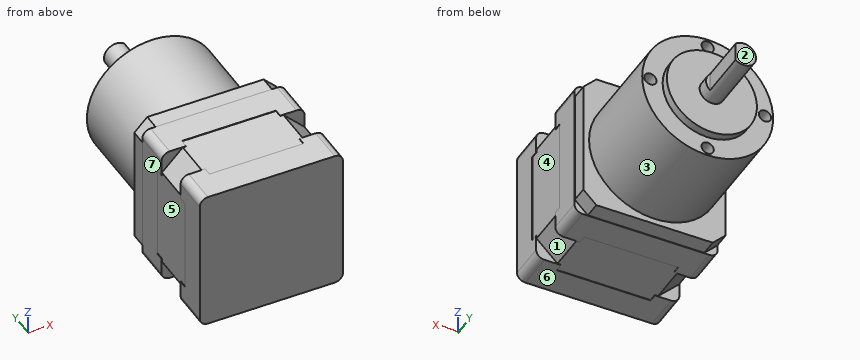
Autodesk Inventor part; units mm, degrees
ref_plane "YZ Plane" through (0, 0, 0) normal (1, 0, 0) x (0, 1, 0)
ref_plane "XZ Plane" through (0, 0, 0) normal (0, 1, 0) x (-1, 0, 0)
ref_plane "XY Plane" through (0, 0, 0) normal (0, 0, 1) x (1, 0, 0)
sketch "Sketch1" plane through (0, 0, 0) normal (0, 1, 0) x (-1, 0, 0)
  circle A0 centre (0, 0) radius 3
  dimension "d0" = 6
extrude "Extrusion1" add sketch "Sketch1" against normal blind 15
sketch "Sketch2" plane through (0, -15, 0) normal (0, -1, 0) x (1, 0, 0)
  circle A0 centre (0, 0) radius 11
  dimension "d3" = 22
extrude "Extrusion2" add sketch "Sketch2" along normal blind 2
sketch "Sketch3" plane through (0, -17, 0) normal (0, -1, 0) x (1, 0, 0)
  circle A0 centre (0, 0) radius 16
  dimension "d6" = 32
extrude "Extrusion3" add sketch "Sketch3" along normal blind 29
sketch "Sketch4" plane through (0, -46, 0) normal (0, -1, 0) x (1, 0, 0)
  line L0 (-17.4, 17.4) -> (17.4, 17.4)
  line L1 (17.4, 17.4) -> (17.4, -17.4)
  line L2 (17.4, -17.4) -> (-17.4, -17.4)
  line L3 (-17.4, -17.4) -> (-17.4, 17.4)
  line L4 (-17.4, 17.4) -> (17.4, -17.4) construction
  line L5 (17.4, 17.4) -> (-17.4, -17.4) construction
  point P0 (0, 0)
  dimension "d9" = 34.8
  dimension "d10" = 34.8
extrude "Extrusion4" add sketch "Sketch4" against normal blind 4
chamfer "Chamfer1" distance 3.175 angle 45 4 edges at (17.4, -44, 17.4) (17.4, -44, -17.4) (-17.4, -44, 17.4) (-17.4, -44, -17.4)
sketch "Sketch5" plane through (0, -46, 0) normal (0, -1, 0) x (1, 0, 0)
  line L0 (17.5, -17.5) -> (-17.5, -17.5)
  line L1 (-17.5, -17.5) -> (-17.5, 17.5)
  line L2 (-17.5, 17.5) -> (17.5, 17.5)
  line L3 (17.5, 17.5) -> (17.5, -17.5)
  line L4 (17.5, -17.5) -> (-17.5, 17.5) construction
  line L5 (-17.5, -17.5) -> (17.5, 17.5) construction
  point P0 (0, 0)
  dimension "d16" = 35
  dimension "d17" = 35
extrude "Extrusion5" add sketch "Sketch5" along normal blind 7
sketch "Sketch6" plane through (0, -53, 0) normal (0, -1, 0) x (1, 0, 0)
  line L0 (-17.5, 17.5) -> (-17.5, -17.5)
  line L1 (-17.5, -17.5) -> (17.5, -17.5)
  line L2 (17.5, -17.5) -> (17.5, 17.5)
  line L3 (17.5, 17.5) -> (-17.5, 17.5)
  line L4 (11.5, 17.5) -> (17.5, 17.5)
  line L5 (17.5, 17.5) -> (17.5, 11.5)
  line L6 (17.5, 11.5) -> (11.5, 11.5)
  line L7 (11.5, 11.5) -> (11.5, 17.5)
  circle A0 centre (0, 0) radius 16
  circle A1 centre (0, 0) radius 16
  line L8 (-17.5, 17.5) -> (-11.5, 17.5)
  line L9 (-17.5, 11.5) -> (-17.5, 17.5)
  line L10 (-11.5, 11.5) -> (-17.5, 11.5)
  line L11 (-11.5, 17.5) -> (-11.5, 11.5)
  line L12 (-17.5, -17.5) -> (-17.5, -11.5)
  line L13 (-11.5, -17.5) -> (-17.5, -17.5)
  line L14 (-11.5, -11.5) -> (-11.5, -17.5)
  line L15 (-17.5, -11.5) -> (-11.5, -11.5)
  line L16 (17.5, -17.5) -> (11.5, -17.5)
  line L17 (17.5, -11.5) -> (17.5, -17.5)
  line L18 (11.5, -11.5) -> (17.5, -11.5)
  line L19 (11.5, -17.5) -> (11.5, -11.5)
  dimension "d43" = 6
  dimension "d44" = 6
  dimension "d47" = 360
extrude "Extrusion6" add sketch "Sketch6" along normal blind 2 contours L3 L11 L10 L0 | L15 L14 L1 L0 | L3 L2 L6 L7 | L19 L18 L2 L1
fillet "Fillet2" radius 2 4 edges at (17.5, -50.5, -17.5) (-17.5, -50.5, -17.5) (-17.5, -50.5, 17.5) (17.5, -50.5, 17.5)
sketch "Sketch7" plane through (0, -53, 0) normal (0, -1, 0) x (1, 0, 0)
  line L0 (-12.2985, -17.4) -> (12.2985, -17.4)
  line L1 (17.4, -12.2985) -> (17.4, 12.2985)
  line L2 (12.2985, 17.4) -> (-12.2985, 17.4)
  line L3 (-17.4, 12.2985) -> (-17.4, -12.2985)
  line L4 (-17.4, -17.4) -> (17.4, 17.4) construction
  line L5 (17.4, -17.4) -> (-17.4, 17.4) construction
  line L6 (-17.4, -12.2985) -> (-12.2985, -17.4)
  line L7 (12.2985, -17.4) -> (17.4, -12.2985)
  line L8 (17.4, 12.2985) -> (12.2985, 17.4)
  line L9 (-12.2985, 17.4) -> (-17.4, 12.2985)
  point P0 (0, 0)
  dimension "d31" = 34.8
  dimension "d32" = 34.8
  dimension "d67" = 42
  dimension "d68" = 42
extrude "Extrusion7" add sketch "Sketch7" along normal blind 6.5
mirror "Mirror1" about plane through (0, -59.5, 0) normal (0, -1, 0) of "Extrusion6", "Extrusion5", "Fillet2", "Extrusion7"
sketch "Sketch8" plane through (0, 0, 0) normal (0, 1, 0) x (1, 0, 0)
  circle A0 centre (0, 0) radius 3
  line L0 (2, 2.2361) -> (2, -2.2361)
  dimension "d50" = 2
extrude "Extrusion8" cut sketch "Sketch8" against normal blind 12 contours A0 L0 picked at (2.1409, -0.5898)
fillet "Fillet3" radius 0.1 1 edges at (2, -12, 0)
sketch "Sketch9" plane through (0, -17, 0) normal (0, 1, 0) x (1, 0, 0)
  circle A0 centre (0, 0) radius 11
  circle A1 centre (0, 0) radius 3
  line L0 (0, 0) -> (0, -14) construction
  circle A2 centre (0, -14) radius 1.5
  dimension "d54" = 14
  dimension "d55" = 3
extrude "Extrusion9" cut sketch "Sketch9" against normal blind 5 contours A2
thread "Thread1"
pattern_circular "Circular Pattern1" count 4 over 360 about axis through (0, -17, 0) along (0, -1, 0) of "Extrusion9"
properties part number "gearedstepper"
Input: part model. Units: mm. Frame: model coordinates. Face numbers are marked on the shaded views. A direction names the side the tool comes from. Round coordinates to 2 decimals unless told otherwise and drop trailing zeros. Loops run counter-clockwise (first coordinate to the right, second up) from the corner with the lowest first, then second, coordinate; pieces in that order, holes last. Notation, with made-up numbers: (-3, 48) -> (21, 48) arc R32 ccw to (21, 76) -> close; hole circle Ø8 at (86, 41.5). An arc over 180 degrees is marked (long way). One line per item, written item: value.
(1) Section C-C (z = 7). Return the cut outline in (x, y).
Geometry check:
outline: (-17.5, -73) -> (17.5, -73) -> (17.5, -66) -> (17.4, -66) -> (17.4, -53) -> (17.5, -53) -> (17.5, -46) -> (17.4, -46) -> (17.4, -42) -> (14.39, -42) -> (14.39, -17) -> (8.49, -17) -> (8.49, -15) -> (-8.49, -15) -> (-8.49, -17) -> (-14.39, -17) -> (-14.39, -42) -> (-17.4, -42) -> (-17.4, -46) -> (-17.5, -46) -> (-17.5, -53) -> (-17.4, -53) -> (-17.4, -66) -> (-17.5, -66) -> close
(2) Pin query (flat end, axial travel): pin 1 (3 mm diameter, centred on y = -44, z = -4.5, fed in from -X); pin 2 (3.5 mm diameter, centred on y = -7, z = 0, fed in from +X); pin 3 (1 mm diameter, centred on y = -18.5, z = 1, fed in from +X). Return the tip coordinate at first contact, or that it passes through.
Geometry check:
pin 1: x = -17.4
pin 2: x = 2
pin 3: x = 15.99
(3) Mould query, pull axis Z, two halves, no side actions, for the marked faces 4, 5, 6 and 7. Classes: pulls with the +Z half, pulls with the -Z half, needs draft (parallel to the pull), parting line crosses it, or undercut.
Geometry check:
face 4: undercut
face 5: undercut
face 6: pulls with the -Z half
face 7: needs draft
(4) Section A-A (y = -62.5). Return the cut outline in (x, z), plus the area to 3 significant figures.
Geometry check:
outline: (-17.4, -12.3) -> (-12.3, -17.4) -> (12.3, -17.4) -> (17.4, -12.3) -> (17.4, 12.3) -> (12.3, 17.4) -> (-12.3, 17.4) -> (-17.4, 12.3) -> close
area: 1,160 mm2
(5) Set-up query: the marked faces 1, 2 and 3. Return all of +Z, -Z, +X, -X, +Y, -Y with unobstructed straight access to the full face (end or side cutting, diameter ignored); none if empty.
Geometry check:
face 1: -Z, +X
face 2: +Z, -Z, +X, -X, +Y
face 3: +Y
(6) Material intervals for line 1 (X direction, y = -18, z = 0); line 2 (Z direction, x = -0.5, y = -35.5), sorted ascending. Write a range as [from, to].
Geometry check:
line 1: [-16, -15.5], [-12.5, 12.5], [15.5, 16]
line 2: [-15.99, 15.99]
(7) Section D-D (y = -31.5). Return the cut outline in (x, z).
Geometry check:
outline: circle Ø32 at (0, 0)
(8) Section B-B (x = 4). Return the cut outline in (y, z).
Geometry check:
outline: (-73, -17.5) -> (-66, -17.5) -> (-66, -17.4) -> (-53, -17.4) -> (-53, -17.5) -> (-46, -17.5) -> (-46, -17.4) -> (-42, -17.4) -> (-42, -15.49) -> (-17, -15.49) -> (-17, -10.25) -> (-15, -10.25) -> (-15, 10.25) -> (-17, 10.25) -> (-17, 15.49) -> (-42, 15.49) -> (-42, 17.4) -> (-46, 17.4) -> (-46, 17.5) -> (-53, 17.5) -> (-53, 17.4) -> (-66, 17.4) -> (-66, 17.5) -> (-73, 17.5) -> close
